from build123d import *

# Parameters (mm, degrees)
SKETCH1_W           = 300
SKETCH1_H           = 192
BOSS_EXTRUDE1_DEPTH = 5
SKETCH2_R           = 1.75
CUT_EXTRUDE1_DEPTH  = 179.160040413
SKETCH4_W           = 46
SKETCH4_H           = 100
CUT_EXTRUDE2_DEPTH  = 179.160040413
SKETCH5_W           = 15
SKETCH5_H           = 55
CUT_EXTRUDE3_DEPTH  = 179.160040413
SKETCH6_R           = 1.6
CUT_EXTRUDE4_DEPTH  = 179.160040413
SKETCH7_W           = 5
SKETCH7_H           = 40
BOSS_EXTRUDE2_DEPTH = 5
SKETCH8_R           = 1.6
CUT_EXTRUDE5_DEPTH  = 183.389692691


with BuildPart() as part:
    # Sketch1 → Boss-Extrude1 (new body)
    with BuildSketch(Plane.XY):
        Rectangle(SKETCH1_W, SKETCH1_H)
    extrude(amount=BOSS_EXTRUDE1_DEPTH)

    # Sketch2 → Cut-Extrude1 (cut, through all)
    with BuildSketch(Plane(origin=(0, 0, 0), x_dir=(-1, 0, 0), z_dir=(0, 0, -1))):
        with Locations((-147.46, 46.46)):
            Circle(SKETCH2_R)
        with Locations((-147.46, -46.46)):
            Circle(SKETCH2_R)
        with Locations((-92.54, 46.46)):
            Circle(SKETCH2_R)
        with Locations((-92.54, -46.46)):
            Circle(SKETCH2_R)
    extrude(amount=-CUT_EXTRUDE1_DEPTH, mode=Mode.SUBTRACT)

    # Sketch4 → Cut-Extrude2 (cut, through all)
    with BuildSketch(Plane.XY.offset(5)):
        with Locations((119.414990718, 0)):
            Rectangle(SKETCH4_W, SKETCH4_H)
    extrude(amount=-CUT_EXTRUDE2_DEPTH, mode=Mode.SUBTRACT)

    # Sketch5 → Cut-Extrude3 (cut, through all)
    with BuildSketch(Plane.XY.offset(5)):
        with BuildLine():
            Line((-70, 42.5), (-130, 42.5))
            ThreePointArc((-130, 42.5), (-131.75, 44.25), (-130, 46))
            Line((-130, 46), (-70, 46))
            ThreePointArc((-70, 46), (-68.25, 44.25), (-70, 42.5))
        make_face()
        with BuildLine():
            Line((-70, -42.5), (-130, -42.5))
            ThreePointArc((-130, -42.5), (-131.75, -44.25), (-130, -46))
            Line((-130, -46), (-70, -46))
            ThreePointArc((-70, -46), (-68.25, -44.25), (-70, -42.5))
        make_face()
        with Locations((-142.5, 0)):
            Rectangle(SKETCH5_W, SKETCH5_H)
    extrude(amount=-CUT_EXTRUDE3_DEPTH, mode=Mode.SUBTRACT)

    # Sketch6 → Cut-Extrude4 (cut, through all)
    with BuildSketch(Plane(origin=(0, 0, 0), x_dir=(-1, 0, 0), z_dir=(0, 0, -1))):
        with Locations((-135, 86)):
            Circle(SKETCH6_R)
        with Locations((-5, 86)):
            Circle(SKETCH6_R)
        with Locations((125, 86)):
            Circle(SKETCH6_R)
        with Locations(Location((125, -86, 0), (0, 0, 180))):
            Circle(SKETCH6_R)
        with Locations(Location((-5, -86, 0), (0, 0, 180))):
            Circle(SKETCH6_R)
        with Locations(Location((-135, -86, 0), (0, 0, 180))):
            Circle(SKETCH6_R)
    extrude(amount=-CUT_EXTRUDE4_DEPTH, mode=Mode.SUBTRACT)

    # Sketch7 → Boss-Extrude2 (add)
    with BuildSketch(Plane(origin=(0, 0, 0), x_dir=(-1, 0, 0), z_dir=(0, 0, -1))):
        with Locations((-152.5, 76)):
            Rectangle(SKETCH7_W, SKETCH7_H)
        with Locations((-152.5, -76)):
            Rectangle(SKETCH7_W, SKETCH7_H)
    extrude(amount=-BOSS_EXTRUDE2_DEPTH)

    # Sketch8 → Cut-Extrude5 (cut, through all)
    with BuildSketch(Plane(origin=(0, 0, 0), x_dir=(-1, 0, 0), z_dir=(0, 0, -1))):
        with Locations((-140, 76.5)):
            Circle(SKETCH8_R)
    extrude(amount=-CUT_EXTRUDE5_DEPTH, mode=Mode.SUBTRACT)


solid = part.part
Geometry check sheet. Reference: the model listing, model coordinates, mm. Round coordinates to 2 decimals unless told otherwise and drop trailing zeros. Order: outer loops, then holes, each group sorted by start corner. A loop starts at its lowest first (then second) coordinate and runs counter-clockwise, first axis right, second up. Notation, with made-up numbers: M 33.5,69.5 L 37.5,69.5 A21 ccw 37.5,76.5 Z; hole C 52.5,74.25 d11. An arc over 180 degrees is marked long. Answer in a Markdown table with one row per item.
(1) Scan lines: probe 1 along X at (y, z) = (-86, 1.65); probe 2 along Y at (x, z) = (135, 1.6); probe 3 along Y at (x, z) = (-103, 3.7). Record each from-to range of solid material in increasing order. Write a range as from..to.
Responses:
| item | result |
|---|---|
| probe 1 | x = -150..-126.6, -123.4..3.4, 6.6..133.4, 136.6..155 |
| probe 2 | y = -96..-87.6, -84.4..-50, 50..84.4, 87.6..96 |
| probe 3 | y = -96..-46, -42.5..42.5, 46..96 |
(2) Sectioned sample at B-B, the plane x = 111. Record the cut outline in (y, z), and give its area (3 significant figures).
Responses:
| item | result |
|---|---|
| outline | M -96,0 L -50,0 L -50,5 L -96,5 Z; M 50,0 L 96,0 L 96,5 L 50,5 Z |
| area | 460 mm² |
(3) Sectioned sample at C-C, the plane z = 3.1. State how many separate pieces and enclosed holes the cut face has, and give its area (3 significant figures).
Responses:
| item | result |
|---|---|
| separate pieces | 1 |
| enclosed holes | 14 |
| area | 52,000 mm² |
(4) Go/stop test with flat-tipped pins: P1, Ø2, axis at y = 17, z = 3, coming from the -X side; P2, Ø3, axis at x = 92.54, y = -46.46, coming from the -Z side; P3, Ø2.5, axis at y = -20, z = 2, coming from the +X side. Record where each tip stops, or that it passes through.
Responses:
| item | result |
|---|---|
| P1 | stops at x = -135 |
| P2 | passes through |
| P3 | stops at x = 150 |
(5) Sectioned sample at A-A, the plane y = 39.5. Record the cut outline in (x, z) (3 decimals).
Responses:
| item | result |
|---|---|
| outline | M -150,0 L 96.415,0 L 96.415,5 L -150,5 Z; M 142.415,0 L 150,0 L 150,5 L 142.415,5 Z |
